```python
from build123d import *

# Parameters (mm, degrees)
SKETCH1_W           = 290
SKETCH1_H           = 400
BOSS_EXTRUDE1_DEPTH = 35
SKETCH2_W           = 270
SKETCH2_H           = 380
CUT_EXTRUDE2_DEPTH  = 10
CUT_EXTRUDE3_DEPTH  = 6
FILLET2_R           = 2
FILLET4_R           = 0.5
FILLET5_R           = 0.5
FILLET6_R           = 0.5
FILLET7_R           = 0.5
FILLET8_R           = 0.5
FILLET9_R           = 0.5


with BuildPart() as part:
    # Sketch1 → Boss-Extrude1 (new body)
    with BuildSketch(Plane(origin=(0, 0, 0), x_dir=(1, 0, 0), z_dir=(0, 1, 0))):
        Rectangle(SKETCH1_W, SKETCH1_H)
    extrude(amount=BOSS_EXTRUDE1_DEPTH)

    # Sketch2 → Cut-Extrude2 (cut)
    with BuildSketch(Plane(origin=(0, 35, 0), x_dir=(1, 0, 0), z_dir=(0, 1, 0))):
        Rectangle(SKETCH2_W, SKETCH2_H)
    extrude(amount=-CUT_EXTRUDE2_DEPTH, mode=Mode.SUBTRACT)

    # Sketch3 → Cut-Extrude3 (cut)
    with BuildSketch(Plane(origin=(0, 25, 0), x_dir=(1, 0, 0), z_dir=(0, 1, 0))):
        with BuildLine():
            Line((-117.13, 185), (-101.75, 185))
            Line((-101.75, 185), (-101.75, 179.7))
            ThreePointArc((-101.75, 179.7), (-95.105829623, 174.14058809), (-99.406157002, 166.62))
            Line((-99.406157002, 166.62), (-99.406157002, 165))
            Line((-99.406157002, 165), (-125.593842998, 165))
            Line((-125.593842998, 165), (-125.593842998, 166.62))
            ThreePointArc((-125.593842998, 166.62), (-129.894170377, 174.14058809), (-123.25, 179.7))
            Line((-123.25, 179.7), (-118.879314151, 179.7))
            Line((-118.879314151, 179.7), (-117.13, 181.5))
            Line((-117.13, 181.5), (-117.13, 185))
        make_face()
    extrude(amount=-CUT_EXTRUDE3_DEPTH, mode=Mode.SUBTRACT)

    # Fillet2
    fillet2_edges = [part.edges().sort_by_distance(p)[0] for p in [
        (-117.13, 22, -181.5),
    ]]
    fillet(fillet2_edges, radius=FILLET2_R)

    # Fillet4
    fillet4_edges = [part.edges().sort_by_distance(p)[0] for p in [
        (-125.593842998, 22, -166.62),
    ]]
    fillet(fillet4_edges, radius=FILLET4_R)

    # Fillet5
    fillet5_edges = [part.edges().sort_by_distance(p)[0] for p in [
        (-99.406157002, 22, -166.62),
    ]]
    fillet(fillet5_edges, radius=FILLET5_R)

    # Fillet6
    fillet6_edges = [part.edges().sort_by_distance(p)[0] for p in [
        (-101.75, 22, -179.7),
    ]]
    fillet(fillet6_edges, radius=FILLET6_R)

    # Fillet7
    fillet7_edges = [part.edges().sort_by_distance(p)[0] for p in [
        (-101.75, 22, -185),
    ]]
    fillet(fillet7_edges, radius=FILLET7_R)

    # Fillet8
    fillet8_edges = [part.edges().sort_by_distance(p)[0] for p in [
        (-117.13, 22, -185),
    ]]
    fillet(fillet8_edges, radius=FILLET8_R)

    # Fillet9
    fillet9_edges = [part.edges().sort_by_distance(p)[0] for p in [
        (-99.406157002, 22, -165),
        (-125.593842998, 22, -165),
    ]]
    fillet(fillet9_edges, radius=FILLET9_R)


solid = part.part
```
Geometry: final body of the model. Coordinates: model frame, mm. A direction names the side the tool comes from. Give positions to 0.01 mm unless a question says otherwise; leave off trailing zeros. Loops run counter-clockwise (first coordinate to the right, second up) from the corner with the lowest first, then second, coordinate; pieces in that order, holes last. Notation, with made-up numbers: (-34.75, 85.25) - (14.25, 85.25) arc R16 cw to (14.25, 90.25) - close; hole circle Ø7 at (3, -27). An arc over 180 degrees is marked (long way). Answer as CSV lines item,"result". Start each with the question number.
(1) Section query A-A (y = 30.5). Output: boundary loops of the cut face in (x, z), and give its area (3 significant figures).
(2) Section query B-B (z = -158). Output: boundary loops of the cut face in (x, y), and give its area (3 significant figures).
(3) Pin query (flat end, axial travel): P1, Ø8, axis at x = 61.5, z = 7, coming from the +Y side; P2, Ø6, axis at x = -104, z = -173.5, coming from the +Y side. Return the tip coordinate at first contact, or that it passes through.
(4) Mould query, pull axis Z, two halves, no side actions, for faces 1 (the face through (-2, 30, 190)), 2 (the face through (-2, 17, -200)), 3 (the face through (-140, 35, -1)), 4 (the face through (-112, 19, -175)). Classes: +Z half, -Z half, draft (parallel to the pull), parting line (faces both ways), or undercut.
(5) Ray query, line 1 along X through (y, z) = (29, -61); line 2 along Y through (x, z) = (-112.5, 26.5). Return the intervals inside material, ascending. Write a range as [from, to].
(6) Reachability of faces 5 (the face through (-145, 17, 3)), 6 (the face through (-2, 30, -190)) from +Z, -Z, +X, -X, +Y, -Y: full face, straight path, thin tool, end or side. Return the list, or none.
(7) Section query C-C (x = 77). Output: boundary loops of the cut face in (y, z), and give its area (3 significant figures).
Worked answers:
1,outline,"(-145, -200) - (145, -200) - (145, 200) - (-145, 200) - close; hole (-135, -190) - (135, -190) - (135, 190) - (-135, 190) - close"
1,area,"13,400 mm^2"
2,outline,"(-145, 0) - (145, 0) - (145, 35) - (135, 35) - (135, 25) - (-135, 25) - (-135, 35) - (-145, 35) - close"
2,area,"7,450 mm^2"
3,P1,"stops at y = 25"
3,P2,"stops at y = 19"
4,face 1,"undercut"
4,face 2,"-Z half"
4,face 3,"draft"
4,face 4,"undercut"
5,line 1,"x = [-145, -135], [135, 145]"
5,line 2,"y = [0, 25]"
6,face 5,"+Z, -Z, -X, +Y, -Y"
6,face 6,"+Y"
7,outline,"(0, -200) - (35, -200) - (35, -190) - (25, -190) - (25, 190) - (35, 190) - (35, 200) - (0, 200) - close"
7,area,"10,200 mm^2"
